```python
from build123d import *

# Parameters (mm, degrees)
F0_W     = 250
F0_H     = 250
F1_DEPTH = 75
F2_W     = 226
F2_H     = 226
F3_DEPTH = 101.6
F4_W     = 226
F4_H     = 13.691548
F5_DEPTH = 75


with BuildPart() as f1:
    # F0 (on Top) → F1 (new body)
    with BuildSketch(Plane.XY):
        Rectangle(F0_W, F0_H)
    extrude(amount=F1_DEPTH)

    # F2 (on face) → F3 (cut)
    with BuildSketch(Plane.XY.offset(75)):
        Rectangle(F2_W, F2_H)
    extrude(amount=-F3_DEPTH, mode=Mode.SUBTRACT)

    # F4 (on face) → F5 (join)
    with BuildSketch(Plane.XY.offset(75)):
        Rectangle(F4_W, F4_H)
    extrude(amount=-F5_DEPTH)


solid = f1.part
```
Geometry: final body of the model. Coordinates: model frame, mm. A direction names the side the tool comes from. Round coordinates to 2 decimals unless told otherwise and drop trailing zeros. Order: outer loops, then holes, each group sorted by start corner. A loop starts at its lowest first (then second) coordinate and runs counter-clockwise, first axis right, second up. Notation, with made-up numbers: M 61,73.5 L 83,73.5 A18 ccw 83,96.5 Z; hole C -35,41.5 d7. An arc over 180 degrees is marked long. Use one line per item in the form item = value. Start each with the question number.
Q1. Mould query, pull axis Y, two halves, no side actions, for faces 1 (the face through (-1, 1, 75)), 2 (the face through (-113, -61, 38)), 3 (the face through (-2, 125, 37)). Classes: +Y half, -Y half, draft (parallel to the pull), parting line (faces both ways), or undercut.
Q2. Cut plane B-B (x = -61). Return loops of the section in (y, z), and give its area (3 significant figures).
Q3. Material intervals for line 1 (Y direction, x = 109, z = 54); line 2 (X direction, y = -75.5, z = 18.5), sorted ascending. Write a range as [from, to].
Q4. Access query for faces 4 (the face through (-125, -2, 37)), 5 (the face through (-2, -6.846, 38)). Directions: +Z, -Z, +X, -X, +Y, -Y. A direction counts if a zero-diameter tool reaches every point of the face in a straight line with its end or side. Return the directions, or none.
Q5. Cut plane A-A (y = -104.5). Return loops of the section in (x, z), and give its area (3 significant figures).
Q6. Cut plane C-C (z = 59). Return loops of the section in (x, y), and give its area (3 significant figures).
Geometry results:
q1.face_1 = draft
q1.face_2 = undercut
q1.face_3 = +Y half
q2.outline = M -125,0 L -113,0 L -113,75 L -125,75 Z; M -6.85,0 L 6.85,0 L 6.85,75 L -6.85,75 Z; M 113,0 L 125,0 L 125,75 L 113,75 Z
q2.area = 2,830 mm^2
q3.line_1 = [-125, -113], [-6.85, 6.85], [113, 125]
q3.line_2 = [-125, -113], [113, 125]
q4.face_4 = +Z, -Z, -X, +Y, -Y
q4.face_5 = +Z, -Z
q5.outline = M -125,0 L -113,0 L -113,75 L -125,75 Z; M 113,0 L 125,0 L 125,75 L 113,75 Z
q5.area = 1,800 mm^2
q6.outline = M -125,-125 L 125,-125 L 125,125 L -125,125 Z; hole M -113,-113 L 113,-113 L 113,-6.85 L -113,-6.85 Z; hole M -113,6.85 L 113,6.85 L 113,113 L -113,113 Z
q6.area = 14,500 mm^2
